Answer from the drawing. Dimensions are ordinates in mm from the lowest x, y and z of the part. A direction names the side the tool comes from. Give positions to 0.01 mm unless a question says otherwise; leave off trailing zeros. Write each loop counter-clockwise with the first axis right and the second up, starting at its lowest first coordinate (ties: lowest second). Pieces come first, ordered by that corner, then holes.
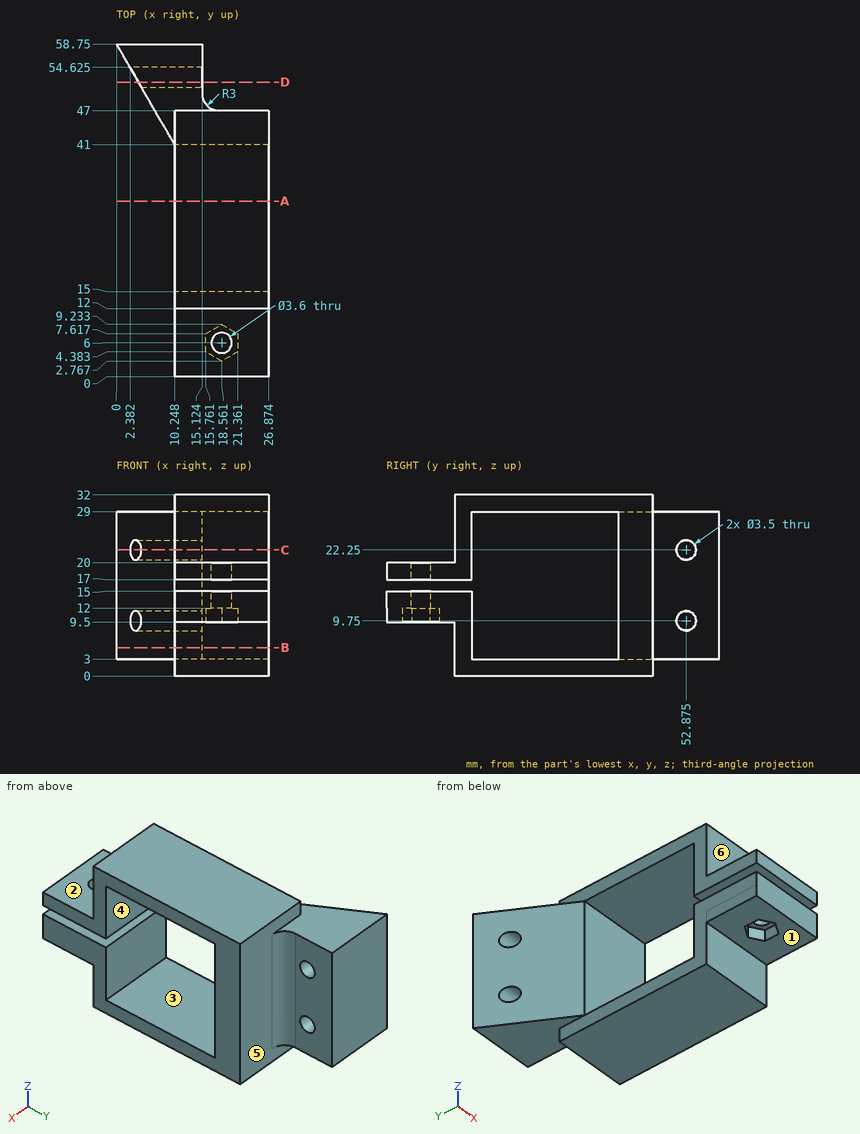
Item 1: Determine the mould class of the marked faces 4, 5 and 6 for opening direction Y: pulls with the +Y half, pulls with the -Y half, needs draft (parallel to the pull), parting line crosses it, or undercut.
Conclusion:
face 4: undercut
face 5: pulls with the +Y half
face 6: pulls with the -Y half
Item 2: A cutting plane is placed at D-D, the plane y = 52. Give the vertices of the cut face in (x, z) (1 decimal), plus the area to 3 significant figures.
Conclusion:
outline: (3.9, 3) - (15.1, 3) - (15.1, 8.2) - (3.9, 8.2) - close; (3.9, 11.3) - (15.1, 11.3) - (15.1, 20.7) - (3.9, 20.7) - close; (3.9, 23.8) - (15.1, 23.8) - (15.1, 29) - (3.9, 29) - close
area: 224 mm2
Item 3: A cutting plane is placed at B-B, the plane z = 5. Give the vertices of the cut face in (x, y).
Conclusion:
outline: (0, 58.75) - (10.25, 41) - (26.87, 41) - (26.87, 47) - (18.12, 47) arc R3 cw to (15.12, 50) - (15.12, 58.75) - close; (10.25, 12) - (26.87, 12) - (26.87, 15) - (10.25, 15) - close
Item 4: A cutting plane is placed at C-C, the plane z = 22.25. Count the separate pieces of the cut face and the enclosed holes in it, plus the area to 3 significant figures.
Conclusion:
separate pieces: 3
enclosed holes: 0
area: 259 mm2
Item 5: Each of these flat-tipped pins is pushed along its axis until it touches: P1, Ø9.5, axis at x = 20.5, z = 24, coming from the +Y side (1 decimal); P2, Ø10, axis at y = 7, z = 17.5, coming from the -X side; P3, Ø1, axis at x = 3, z = 5.5, coming from the -Y side. Where does it stop, or does it pass through?
Conclusion:
P1: stops at y = 48.2
P2: stops at x = 10.25
P3: stops at y = 52.69
Item 6: A cutting plane is placed at A-A, the plane y = 31. Give the vertices of the cut face in (x, z).
Conclusion:
outline: (10.25, 0) - (26.87, 0) - (26.87, 3) - (10.25, 3) - close; (10.25, 29) - (26.87, 29) - (26.87, 32) - (10.25, 32) - close
Item 7: Consider probe 1 along Z at (x, y) = (21.5, 39); probe 2 along Y at (x, z) = (14.5, 26.5); probe 3 along Z at (x, y) = (15, 6.5). Determine where each line is inside the solid, lowest interval first.
Conclusion:
probe 1: z = 0 to 3, 29 to 32
probe 2: y = 12 to 15, 41 to 58.75
probe 3: z = 9.5 to 15, 17 to 20
Item 8: Which of the six approach directions +Z, -Z, +X, -X, +Y, -Y give full straight-line access (tool end or side, diameter ignored) to the marked faces 1, 2 and 3?
Conclusion:
face 1: -Z, +X, -X, -Y
face 2: +Z, +X, -X, -Y
face 3: +X, -X
